Build history of the part. All positions in model axes, mm. A direction names the side the tool comes from. Round coordinates to 2 decimals unless told otherwise and drop trailing zeros. Loops run counter-clockwise (first coordinate to the right, second up) from the corner with the lowest first, then second, coordinate; pieces in that order, holes last. Notation, with made-up numbers: M 12,-13 L 35,-13 A33 cw 35,21 Z; hole C 64,-1 d2. An arc over 180 degrees is marked long. Use one line per item in the form item = value. Start each with the question number.
```python
from build123d import *

# Parameters (mm, degrees)
CIRPATTERN2_COUNT                = 3
CIRPATTERN1_COUNT                = 6
F_8_32_TAPPED_HOLE1_D            = 3.4544
F_8_32_TAPPED_HOLE1_DEPTH        = 6.35
F_8_32_TAPPED_HOLE1_TIP          = 1.037806461
F_50_0_07_DIAMETER_HOLE1_D       = 1.778
F_50_0_07_DIAMETER_HOLE1_DEPTH   = 11.938
F_50_0_07_DIAMETER_HOLE1_TIP     = 0.53416509
Q_0_332_DIAMETER_HOLE1_D         = 8.4328
F_3_8_0_375_DIAMETER_HOLE1_D     = 9.525
F_3_8_0_375_DIAMETER_HOLE1_DEPTH = 9.144
F_3_8_0_375_DIAMETER_HOLE1_TIP   = 2.861598698


with BuildPart() as part:
    # Sketch1 → Revolve1 (revolve)
    with BuildSketch(Plane.XY, mode=Mode.PRIVATE) as revolve1_sk:
        Polygon((-12.599, 0), (0, 0), (0, 34.8361), (-2.54, 34.8361), (-2.54, 32.7406), (-6.223, 32.7406), (-6.223, 34.8361), (-8.763, 34.8361), (-8.763, 32.7406), (-12.446, 32.7406), (-12.446, 34.8361), (-14.885, 34.8361), (-14.885, 29.1592), (-18.06, 29.1592), (-18.06, 4.7625), (-12.599, 4.7625), align=None)
    revolve(revolve1_sk.sketch.rotate(Axis((17.779879847, 0, 0), (-1, 0, 0)), 90), axis=Axis((17.779879847, 0, 0), (-1, 0, 0)))

    # Sketch24 → 20 _0.161_ Diameter Hole1 (revolve, cut)
    with BuildSketch(Plane(origin=(-18.06, 22.225, 0), x_dir=(0, 0, 1), z_dir=(0, 1, 0))):
        Polygon((0, 0), (0, 10.880579708), (2.0447, 9.652), (2.0447, 0), align=None)
    f_20_0_161_diameter_hole1 = revolve(axis=Axis((-24.41, 22.225, 0), (1, 0, 0)), mode=Mode.SUBTRACT)

    # CirPattern2: 20 _0.161_ Diameter Hole1 ×3 about axis
    cirpattern2_axis = Axis((0, 0, 0), (1, 0, 0))
    for i in range(1, CIRPATTERN2_COUNT):
        add(f_20_0_161_diameter_hole1.rotate(cirpattern2_axis, i * 360 / CIRPATTERN2_COUNT), mode=Mode.SUBTRACT)

    # Sketch19 → 1.5 _1.5_ Diameter Hole4 (revolve, cut)
    with BuildSketch(Plane(origin=(0.866676253, -0.068634017, -6.358122396), x_dir=(0.15097729062415485, 0.7033639629103843, -0.6946113973977026), z_dir=(-0.040958510327058266, 0.7065134112073841, 0.7065134112073841))):
        Polygon((0, 0), (0, 24.51962842), (0.75, 24.068982956), (0.75, 0), align=None)
    f_1_5_1_5_diameter_hole4 = revolve(axis=Axis((7.138497216, -0.565313443, -5.497848394), (-0.9876883405951382, 0.07821723252011407, -0.13547622075226584)), mode=Mode.SUBTRACT)

    # CirPattern1: 1.5 _1.5_ Diameter Hole4 ×6 about axis
    cirpattern1_axis = Axis((-26.67, 0, 0), (1, 0, 0))
    for i in range(1, CIRPATTERN1_COUNT):
        add(f_1_5_1_5_diameter_hole4.rotate(cirpattern1_axis, i * 360 / CIRPATTERN1_COUNT), mode=Mode.SUBTRACT)

    # 8-32 Tapped Hole1
    with Locations(Plane.ZY.offset(12.599)):
        with Locations((0, 0)):
            Hole(F_8_32_TAPPED_HOLE1_D / 2, depth=F_8_32_TAPPED_HOLE1_DEPTH)
            with Locations((0, 0, -(F_8_32_TAPPED_HOLE1_DEPTH + F_8_32_TAPPED_HOLE1_TIP / 2))):  # 118° drill point
                Cone(0, F_8_32_TAPPED_HOLE1_D / 2, F_8_32_TAPPED_HOLE1_TIP, mode=Mode.SUBTRACT)

    # 50 _0.07_ Diameter Hole1
    with Locations(Plane.ZY.offset(18.06)):
        with Locations((19.632362891, 11.33475)):
            Hole(F_50_0_07_DIAMETER_HOLE1_D / 2, depth=F_50_0_07_DIAMETER_HOLE1_DEPTH)
            with Locations((0, 0, -(F_50_0_07_DIAMETER_HOLE1_DEPTH + F_50_0_07_DIAMETER_HOLE1_TIP / 2))):  # 118° drill point
                Cone(0, F_50_0_07_DIAMETER_HOLE1_D / 2, F_50_0_07_DIAMETER_HOLE1_TIP, mode=Mode.SUBTRACT)

    # Q _0.332_ Diameter Hole1 (through all)
    with Locations(Plane.ZY.offset(18.06)):
        with Locations((0, -22.225)):
            Hole(Q_0_332_DIAMETER_HOLE1_D / 2)

    # 3_8 _0.375_ Diameter Hole1
    with Locations(Plane(origin=(0, 0, 0), x_dir=(0, 0, -1), z_dir=(1, 0, 0))):
        with Locations((0, -22.225)):
            Hole(F_3_8_0_375_DIAMETER_HOLE1_D / 2, depth=F_3_8_0_375_DIAMETER_HOLE1_DEPTH)
            with Locations((0, 0, -(F_3_8_0_375_DIAMETER_HOLE1_DEPTH + F_3_8_0_375_DIAMETER_HOLE1_TIP / 2))):  # 118° drill point
                Cone(0, F_3_8_0_375_DIAMETER_HOLE1_D / 2, F_3_8_0_375_DIAMETER_HOLE1_TIP, mode=Mode.SUBTRACT)


solid = part.part
```
Q1. Saw through at B-B (y = 19). Give the cut face in (x, z) (3 decimals).
Q2. Pull direction Y, two halves, no side cores. Call faces 1 (the face through (-7.511, -29.374, -18.728)), 2 (the face through (-18.06, 6, 0)), 3 (the face through (-13.706, -18.044, 0.549)): pulls with the +Y half, pulls with the -Y half, needs draft (parallel to the pull), parting line crosses it, or undercut.
Q3. Drop flat-ended pins along their axis: P1, Ø2.5, axis at y = 22.225, z = 0, coming from the -X side; P2, Ø3, axis at y = 17, z = 3.5, coming from the +X side; P3, Ø8, axis at x = -6, z = 3, coming from the +Y side; P4, Ø2, axis at y = 0, z = 0, coming from the -X side. Give the stop position or say it passes through.
Q4. Wall check: probe 1 along Y at (x, z) = (-15, 0); probe 2 along Z at (x, y) = (-16.75, -2); probe 3 along X at (y, z) = (-11.5, -29.5) (3 decimals). Give the ranges that are in metal, low to high.
Q5. Tool access for faces 4 (the face through (-13.3, 24.22, -0.44)), 5 (the face through (0, 0, 0)), 6 (the face through (-4.6, -17.5, -0.6)), 7 (the face through (-10.63, -32.462, 4.262)): list every direction of +Z, -Z, +X, -X, +Y, -Y with a clear straight run to the whole face (end or side of a thin tool).
Q6. Saw through at C-C (x = -16). Give the number of separate pieces and of enclosed holes in the cut face, and give its area (3 significant figures).
Q7. Saw through at A-A (z = 22.5). Give the cut face in (x, y) (3 decimals).
Filled in:
q1.outline = M -18.06,-22.119 L -14.885,-22.119 L -14.885,-29.199 L -12.446,-29.199 L -12.446,-26.664 L -8.763,-26.664 L -8.763,-29.199 L -6.223,-29.199 L -6.223,-26.664 L -2.54,-26.664 L -2.54,-29.199 L 0,-29.199 L 0,29.199 L -2.54,29.199 L -2.54,26.664 L -6.223,26.664 L -6.223,29.199 L -8.763,29.199 L -8.763,26.664 L -12.446,26.664 L -12.446,29.199 L -14.885,29.199 L -14.885,22.119 L -18.06,22.119 Z
q2.face_1 = parting line crosses it
q2.face_2 = needs draft
q2.face_3 = undercut
q3.P1 = -7.93
q3.P2 = 0
q3.P3 = 34.84
q3.P4 = -5.81
q4.probe_1 = -29.16 to -26.44, -18.01 to -4.76, 4.76 to 20.18, 24.27 to 29.16
q4.probe_2 = -29.09 to -4.32, 4.32 to 8.44, 9.12 to 29.09
q4.probe_3 = -14.885 to 0
q5.face_4 = -X
q5.face_5 = +Z, -Z, +X, +Y, -Y
q5.face_6 = +X
q5.face_7 = none
q6.separate_pieces = 1
q6.enclosed_holes = 12
q6.area = 2,490 mm²
q7.outline = M -18.06,-18.547 L -14.885,-18.547 L -14.885,-26.595 L -12.446,-26.595 L -12.446,-23.784 L -8.763,-23.784 L -8.763,-26.595 L -6.223,-26.595 L -6.223,-23.784 L -2.54,-23.784 L -2.54,-26.595 L 0,-26.595 L 0,26.595 L -2.54,26.595 L -2.54,23.784 L -6.223,23.784 L -6.223,26.595 L -8.763,26.595 L -8.763,23.784 L -12.446,23.784 L -12.446,26.595 L -14.885,26.595 L -14.885,18.547 L -18.06,18.547 Z
